```python
from build123d import *

# Parameters (mm, degrees)
EXTRUDE_1_DEPTH     = 12.4
SKETCH_2_R          = 17.5
CUT_EXTRUDE_1_DEPTH = 7
SKETCH_3_R          = 11
CUT_EXTRUDE_2_DEPTH = 61.510329697
SKETCH_4_R          = 3.25
SKETCH_4_R_2        = 1.525
CUT_EXTRUDE_3_DEPTH = 10
SKETCH_4_3_R        = 1.525
SKETCH_4_3_R_2      = 1.75
CUT_EXTRUDE_4_DEPTH = 62.36986231


with BuildPart() as part:
    # Sketch 1 → Extrude 1 (new body)
    with BuildSketch(Plane(origin=(0, 0, 0), x_dir=(1, 0, 0), z_dir=(0, 1, 0))):
        Polygon((0, 40.025126266), (0, 2.474873734), (2.474873734, 0), (40.025126266, 0), (42.5, 2.474873734), (42.5, 40.025126266), (40.025126266, 42.5), (2.474873734, 42.5), align=None)
    extrude(amount=EXTRUDE_1_DEPTH)

    # Sketch 2 → Cut-Extrude 1 (cut)
    with BuildSketch(Plane(origin=(0, 12.4, 0), x_dir=(1, 0, 0), z_dir=(0, 1, 0))):
        with Locations(Location((21.25, 21.25, 0), (0, 0, 270))):
            Circle(SKETCH_2_R)
    extrude(amount=-CUT_EXTRUDE_1_DEPTH, mode=Mode.SUBTRACT)

    # Sketch 3 → Cut-Extrude 2 (cut, through all)
    with BuildSketch(Plane(origin=(0, 5.4, 0), x_dir=(1, 0, 0), z_dir=(0, 1, 0))):
        with Locations(Location((21.25, 21.25, 0), (0, 0, 270))):
            Circle(SKETCH_3_R)
    extrude(amount=-CUT_EXTRUDE_2_DEPTH, mode=Mode.SUBTRACT)

    # Sketch 4 → Cut-Extrude 3 (cut)
    with BuildSketch(Plane(origin=(0, 12.4, 0), x_dir=(1, 0, 0), z_dir=(0, 1, 0))):
        with Locations(Location((5.75, 5.75, 0), (0, 0, 270))):
            Circle(SKETCH_4_R)
        with Locations(Location((36.75, 36.75, 0), (0, 0, 270))):
            Circle(SKETCH_4_R)
        with Locations((5.75, 5.75)):
            Circle(SKETCH_4_R_2)
        with Locations((36.75, 36.75)):
            Circle(SKETCH_4_R_2)
    extrude(amount=-CUT_EXTRUDE_3_DEPTH, mode=Mode.SUBTRACT)

    # Sketch 4_3 → Cut-Extrude 4 (cut, through all)
    with BuildSketch(Plane(origin=(0, 12.4, 0), x_dir=(1, 0, 0), z_dir=(0, 1, 0))):
        with Locations(Location((5.75, 5.75, 0), (0, 0, 270))):
            Circle(SKETCH_4_3_R)
        with Locations(Location((38.92766953, 3.57233047, 0), (0, 0, 270))):
            Circle(SKETCH_4_3_R_2)
        with Locations(Location((36.75, 36.75, 0), (0, 0, 270))):
            Circle(SKETCH_4_3_R)
        with Locations(Location((3.57233047, 38.92766953, 0), (0, 0, 270))):
            Circle(SKETCH_4_3_R_2)
    extrude(amount=-CUT_EXTRUDE_4_DEPTH, mode=Mode.SUBTRACT)


solid = part.part
```
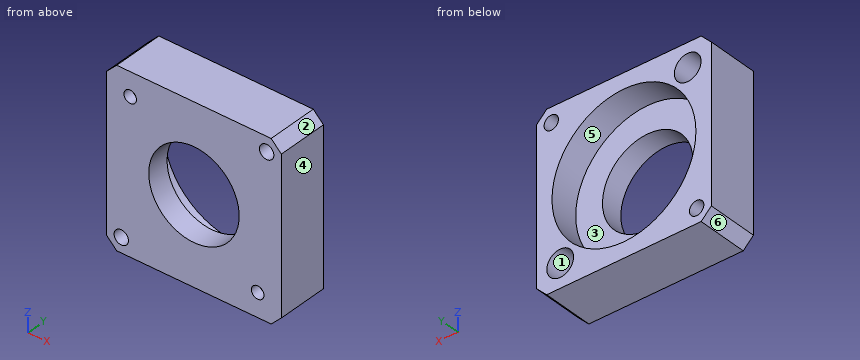
The listing builds one solid part. Answer for the finished solid, in the listing's coordinates (mm). Face numbers are marked on the shaded views. A direction names the side the tool comes from. Round coordinates to 2 decimals unless told otherwise and drop trailing zeros. Loops run counter-clockwise (first coordinate to the right, second up) from the corner with the lowest first, then second, coordinate; pieces in that order, holes last. Notation, with made-up numbers: (68, 21.5) - (91, 21.5) arc R17 ccw to (91, 26.5) - close; hole circle Ø1 at (-6.5, 22). An arc over 180 degrees is marked (long way). Use one line per item in the form item = value. Start each with the question number.
1. Given pin 1 Ø21 at (x, z) = (21.25, -21.25) entering from +Y; pin 2 Ø3 at (x, z) = (6, -7) entering from +Y, each flat-ended and moving along its own axis, determine where each tip first touches the part or whether it passes through.
2. The part is cut by section A-A on z = -21.25. Determine the outline of the cut face in (x, y), then the cut area to 3 significant figures.
3. A tool of negligible diameter and unlimited length cuts with its end or side. For the marked faces 1 and 2, from which of +Z, -Z, +X, -X, +Y, -Y can it reach the whole face along a straight path? Write none if from no direction.
4. The part is cut by section C-C on y = 3. Determine the outline of the cut face in (x, z), then the cut area to 3 significant figures.
5. The part is cut by section D-D on z = -36. Determine the outline of the cut face in (x, y).
6. Consider line 1 (X direction, y = 1.9, z = -36.75) (3 decimals); line 2 (X direction, y = 9, z = -6.5); line 3 (X direction, y = 3.9, z = -21.25). Determine where each line is inside the solid, lowest interval first. Write a range as [from, to].
7. The part is cut by section B-B on x = 21.25. Determine the outline of the cut face in (y, z), then the cut area to 3 significant figures.
8. For a pull along X with two mould halves and no side action, classify the marked faces 3, 4, 5 and 6 as pulls with the +X half, pulls with the -X half, needs draft (parallel to the pull), parting line crosses it, or undercut.
Geometry check:
q1.pin_1 = through
q1.pin_2 = 2.4
q2.outline = (0, 0) - (10.25, 0) - (10.25, 5.4) - (3.75, 5.4) - (3.75, 12.4) - (0, 12.4) - close; (32.25, 0) - (42.5, 0) - (42.5, 12.4) - (38.75, 12.4) - (38.75, 5.4) - (32.25, 5.4) - close
q2.area = 163 mm^2
q3.face_1 = +Y
q3.face_2 = +Z, +X, +Y, -Y
q4.outline = (0, -40.03) - (2.47, -42.5) - (40.03, -42.5) - (42.5, -40.03) - (42.5, -2.47) - (40.03, 0) - (2.47, 0) - (0, -2.47) - close; hole circle Ø3.5 at (3.57, -38.93); hole circle Ø6.5 at (5.75, -5.75); hole circle Ø22 at (21.25, -21.25); hole circle Ø6.5 at (36.75, -36.75); hole circle Ø3.5 at (38.93, -3.57)
q4.area = 1,330 mm^2
q5.outline = (0, 0) - (35.42, 0) - (35.42, 2.4) - (33.59, 2.4) - (33.59, 12.4) - (30.67, 12.4) - (30.67, 5.4) - (11.83, 5.4) - (11.83, 12.4) - (0, 12.4) - close; (38.08, 0) - (42.5, 0) - (42.5, 12.4) - (39.91, 12.4) - (39.91, 2.4) - (38.08, 2.4) - close
q6.line_1 = [0, 35.225], [38.275, 42.5]
q6.line_2 = [0, 2.59], [8.91, 11.83], [30.67, 42.5]
q6.line_3 = [0, 10.25], [32.25, 42.5]
q7.outline = (0, -42.5) - (12.4, -42.5) - (12.4, -38.75) - (5.4, -38.75) - (5.4, -32.25) - (0, -32.25) - close; (0, -10.25) - (5.4, -10.25) - (5.4, -3.75) - (12.4, -3.75) - (12.4, 0) - (0, 0) - close
q7.area = 163 mm^2
q8.face_3 = undercut
q8.face_4 = pulls with the +X half
q8.face_5 = undercut
q8.face_6 = pulls with the -X half
